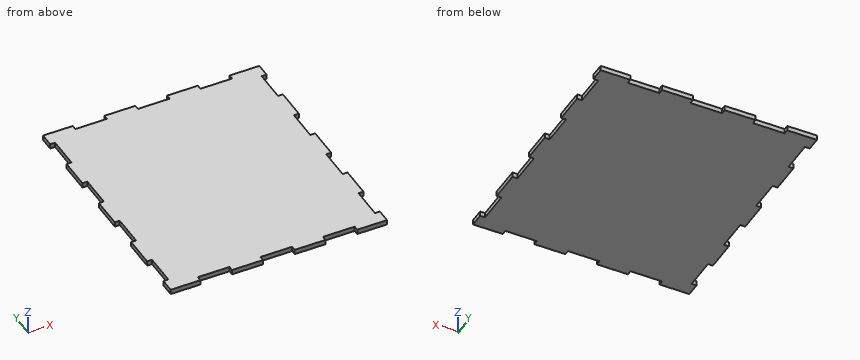
```python
from build123d import *

# Parameters (mm, degrees)
SKETCH1_W           = 140
SKETCH1_H           = 160
BOSS_EXTRUDE1_DEPTH = 3.175
SKETCH2_W           = 3.175
SKETCH2_H           = 20.5
SKETCH2_W_2         = 20.5
SKETCH2_H_2         = 3.175
CUT_EXTRUDE1_DEPTH  = 3.175


with BuildPart() as part:
    # Sketch1 → Boss-Extrude1 (new body)
    with BuildSketch(Plane.XY):
        with Locations((5.981871877, 80)):
            Rectangle(SKETCH1_W, SKETCH1_H)
    extrude(amount=BOSS_EXTRUDE1_DEPTH)

    # Sketch2 → Cut-Extrude1 (cut)
    with BuildSketch(Plane.XY.offset(3.175)):
        with Locations((-62.430628123, 19.25)):
            Rectangle(SKETCH2_W, SKETCH2_H)
        with Locations((-62.430628123, 59.75)):
            Rectangle(SKETCH2_W, SKETCH2_H)
        with Locations((-62.430628123, 100.25)):
            Rectangle(SKETCH2_W, SKETCH2_H)
        with Locations((-62.430628123, 140.75)):
            Rectangle(SKETCH2_W, SKETCH2_H)
        with Locations((-34.518128123, 158.4125)):
            Rectangle(SKETCH2_W_2, SKETCH2_H_2)
        with Locations((5.981871877, 158.4125)):
            Rectangle(SKETCH2_W_2, SKETCH2_H_2)
        with Locations((46.481871877, 158.4125)):
            Rectangle(SKETCH2_W_2, SKETCH2_H_2)
        with Locations((74.394371877, 140.75)):
            Rectangle(SKETCH2_W, SKETCH2_H)
        with Locations((74.394371877, 100.25)):
            Rectangle(SKETCH2_W, SKETCH2_H)
        with Locations((74.394371877, 59.75)):
            Rectangle(SKETCH2_W, SKETCH2_H)
        with Locations((74.394371877, 19.25)):
            Rectangle(SKETCH2_W, SKETCH2_H)
        with Locations((46.481871877, 1.5875)):
            Rectangle(SKETCH2_W_2, SKETCH2_H_2)
        with Locations((5.981871877, 1.5875)):
            Rectangle(SKETCH2_W_2, SKETCH2_H_2)
        with Locations((-34.518128123, 1.5875)):
            Rectangle(SKETCH2_W_2, SKETCH2_H_2)
    extrude(amount=-CUT_EXTRUDE1_DEPTH, mode=Mode.SUBTRACT)


solid = part.part
```
Could you check a few things on this model? Use its own coordinates, in mm. Give positions to 0.01 mm unless a question says otherwise; leave off trailing zeros. Loops run counter-clockwise (first coordinate to the right, second up) from the corner with the lowest first, then second, coordinate; pieces in that order, holes last. Notation, with made-up numbers: (-19, -23) -> (-3, -23) arc R24 ccw to (-3, 4) -> close; hole circle Ø1 at (83.5, 34). An arc over 180 degrees is marked (long way). Put each result on its own line as item: value.
(1) Imagine slicing it at A-A on y = 27. Write out the boundary of the cut face in (x, z) (3 decimals).
Computed:
outline: (-60.843, 0) -> (72.807, 0) -> (72.807, 3.175) -> (-60.843, 3.175) -> close
(2) Imagine slicing it at B-B on x = 54.5. Write out the boundary of the cut face in (y, z) (3 decimals), plus the area to 3 significant figures.
Computed:
outline: (3.175, 0) -> (156.825, 0) -> (156.825, 3.175) -> (3.175, 3.175) -> close
area: 488 mm^2
(3) I'm going to push a flat-ended pin straight in: pin 1 Ø1.5 at (y, z) = (22, 0.5) entering from -X. Where does the tip first touch, or does it pass through?
Computed:
pin 1: x = -60.84
(4) Please list where these lines run through material, in increasing order: probe 1 along Y at (x, z) = (54.5, 1.6) (3 decimals); probe 2 along X at (y, z) = (16, 0.55). Write a range as [from, to].
Computed:
probe 1: [3.175, 156.825]
probe 2: [-60.84, 72.81]
